Geometry check sheet. Reference: the model listing, model coordinates, mm. A direction names the side the tool comes from. Round coordinates to 2 decimals unless told otherwise and drop trailing zeros. Loops run counter-clockwise (first coordinate to the right, second up) from the corner with the lowest first, then second, coordinate; pieces in that order, holes last. Notation, with made-up numbers: (-13.5, 27.25) - (37.5, 27.25) arc R29 cw to (37.5, 62.25) - close; hole circle Ø9 at (30.5, -34). An arc over 180 degrees is marked (long way). Write item = value, one per line.
```python
from build123d import *

# Parameters (mm, degrees)
EXTRUDE_1_DEPTH             = 20
FILLET_1_R                  = 2
FILLET_2_R                  = 2
CUT_EXTRUDE_2_DEPTH         = 10
SKETCH_34_R                 = 3.25
CUT_EXTRUDE_3_DEPTH         = 6
HOLE_WIZARD_M4_2_D          = 3.3
HOLE_WIZARD_M4_2_DEPTH      = 4
SKETCH_38_W                 = 5
SKETCH_38_H                 = 10
CUT_EXTRUDE_4_DEPTH         = 11
SKETCH_40_W                 = 1.65
SKETCH_40_H                 = 8
HOLE_WIZARD_M4_3_AT_2_COUNT = 2
HOLE_WIZARD_M4_3_AT_2_PITCH = 10
CUT_EXTRUDE_5_DEPTH         = 4.5


with BuildPart() as part:
    # 草图1 → 凸台-拉伸1 (new body)
    with BuildSketch(Plane.XY):
        Polygon((0.020144186, -0.052366179), (0.016918395, 5.947632954), (-19.983081605, 5.947632954), (-20.000068427, 12.447632954), (0.03759791, 12.447632954), (0.03759791, 20.447632954), (-19.96240209, 20.447632954), (-11.597239053, 51.666846423), (-21.256497316, 54.255036874), (-30.315163894, 20.447632954), (-30.279663837, -0.052366179), align=None)
    extrude(amount=EXTRUDE_1_DEPTH)

    # 圆角1
    fillet_1_edges = [part.edges().sort_by_distance(p)[0] for p in [
        (-19.96240209, 20.447632954, 10),
    ]]
    fillet(fillet_1_edges, radius=FILLET_1_R)

    # 圆角2
    fillet_2_edges = [part.edges().sort_by_distance(p)[0] for p in [
        (-30.279663837, -0.052366179, 10),
    ]]
    fillet(fillet_2_edges, radius=FILLET_2_R)

    # 草图33 → 切除-拉伸2 (cut)
    with BuildSketch(Plane.XY.offset(20)):
        Polygon((-21.256497316, 54.255036874), (-11.597239053, 51.666846423), (-14.185429504, 42.00758816), (-23.844687767, 44.595778611), align=None)
    extrude(amount=-CUT_EXTRUDE_2_DEPTH, mode=Mode.SUBTRACT)

    # 草图34 → 切除-拉伸3 (cut)
    with BuildSketch(Plane(origin=(0, 0, 0), x_dir=(-1, 0, 0), z_dir=(0, 0, -1))):
        with Locations((17.72096341, 48.131312517)):
            Circle(SKETCH_34_R)
    extrude(amount=-CUT_EXTRUDE_3_DEPTH, mode=Mode.SUBTRACT)

    # M4 螺纹孔的螺纹孔钻头2
    with Locations(Plane(origin=(0, 0, 6), x_dir=(-1, 0, 0), z_dir=(0, 0, -1))):
        with Locations((17.72096341, 48.131312517)):
            Hole(HOLE_WIZARD_M4_2_D / 2, depth=HOLE_WIZARD_M4_2_DEPTH)

    # 草图38 → 切除-拉伸4 (cut)
    with BuildSketch(Plane(origin=(-23.737082949, 6.360332207, 0), x_dir=(0, 0, -1), z_dir=(0.965925826, -0.258819045, 0))):
        with Locations((-2.5, 41.904754985)):
            Rectangle(SKETCH_38_W, SKETCH_38_H)
    extrude(amount=-CUT_EXTRUDE_4_DEPTH, mode=Mode.SUBTRACT)

    # 草图40 → M4 螺纹孔的螺纹孔钻头3 (revolve, cut)
    with BuildSketch(Plane(origin=(-5.798619526, 12.447632954, 5), x_dir=(0, 0, -1), z_dir=(1, 0, 0))):
        with Locations((0.825, 4)):
            Rectangle(SKETCH_40_W, SKETCH_40_H)
    hole_wizard_m4_3 = revolve(axis=Axis((-5.798619526, 6.097632954, 5), (0, 1, 0)), mode=Mode.SUBTRACT)

    # M4 螺纹孔的螺纹孔钻头3 at 2: M4 螺纹孔的螺纹孔钻头3 ×2
    with Locations(*[(0, 0, i * HOLE_WIZARD_M4_3_AT_2_PITCH) for i in range(1, HOLE_WIZARD_M4_3_AT_2_COUNT)]):
        add(hole_wizard_m4_3, mode=Mode.SUBTRACT)

    # 草图41 → 切除-拉伸5 (cut)
    with BuildSketch(Plane.XZ.offset(-12.447632954)):
        with BuildLine():
            Line((-7.265759602, 12.1), (-4.331479451, 12.1))
            ThreePointArc((-4.331479451, 12.1), (-2.548619526, 15), (-4.331479451, 17.9))
            Line((-4.331479451, 17.9), (-7.265759602, 17.9))
            ThreePointArc((-7.265759602, 17.9), (-9.048619526, 15), (-7.265759602, 12.1))
        make_face()
        with BuildLine():
            Line((-7.265759602, 2.1), (-4.331479451, 2.1))
            ThreePointArc((-4.331479451, 2.1), (-2.548619526, 5), (-4.331479451, 7.9))
            Line((-4.331479451, 7.9), (-7.265759602, 7.9))
            ThreePointArc((-7.265759602, 7.9), (-9.048619526, 5), (-7.265759602, 2.1))
        make_face()
    extrude(amount=-CUT_EXTRUDE_5_DEPTH, mode=Mode.SUBTRACT)


solid = part.part
```
(1) Section check B-B (x = -18). Enter the section's corners in (y, z).
Answers follow:
outline = (-0.05, 0) - (5.95, 0) - (5.95, 20) - (-0.05, 20) - close; (12.45, 0) - (20.55, 0) - (20.55, 20) - (12.45, 20) - close; (27.77, 0) - (43.03, 0) - (43.03, 5) - (44.89, 5) - (44.89, 6) - (46.51, 6) - (46.51, 10) - (43.03, 10) - (43.03, 20) - (27.77, 20) - close; (49.76, 6) - (51.37, 6) - (51.37, 5) - (53.38, 5) - (53.38, 10) - (49.76, 10) - close
(2) Scan lines: L1, parallel to Z at x = -5, y = 13.5; L2, parallel to Y at x = -6, z = 9.75; L3, parallel to X at y = 18.65, z = 15. Record each from-to range of solid material in increasing order. Write a range as [from, to].
Answers follow:
L1 = [0, 2.1], [7.9, 12.1], [17.9, 20]
L2 = [-0.05, 5.95], [12.45, 20.45]
L3 = [-30.31, -7.45], [-4.15, 0.04]
(3) Mould release check, pull along Y, two halves, no side actions. Record for faces 5 (the flat face through (-6, 16.948, 13)), 6 (the flat face through (-19, 18, 20)), 7 (the flat face through (-16.359, 52.943, 7.465)): pulls with the +Y half, pulls with the -Y half, needs draft (parallel to the pull), parting line crosses it, or undercut.
Answers follow:
face_5 = undercut
face_6 = needs draft
face_7 = pulls with the +Y half
(4) Set-up check for faces 1 (the cylindrical face through (-6.91, 18.72, 6.22)), 2 (the flat face through (-14, 47, 5)), 3 (the cylindrical face through (-2.55, 14.67, 14.95)), 4 (the flat face through (-9, 20.448, 10)): record each of +Z, -Z, +X, -X, +Y, -Y from which the full face is reachable in a straight line by a thin tool's end or side.
Answers follow:
face_1 = +Y
face_2 = -Z, +X, +Y
face_3 = none
face_4 = +Z, -Z, +X
(5) Gauge pin test, flat ends, axial feed: pin 1 (5 mm diameter, centred on y = 30.5, z = 10.5, fed in from -X); pin 2 (2 mm diameter, centred on x = -17, z = 11.5, fed in from +Y); pin 3 (3 mm diameter, centred on x = -16, y = 49, fed in from -Z); pin 4 (3 mm diameter, centred on x = -17.72, y = 48.13, fed in from +Z). Record the tip position at first contact, or that the pin passes through.
Answers follow:
pin_1 = -28.29
pin_2 = 43.03
pin_3 = 5
pin_4 = through
(6) Section check A-A (z = 15). Enter the section's corners in (x, y).
Answers follow:
outline = (-30.32, 20.45) - (-30.28, 1.94) arc R2 ccw to (-28.28, -0.05) - (0.02, -0.05) - (0.02, 5.95) - (-19.98, 5.95) - (-20, 12.45) - (-9.05, 12.45) - (-9.05, 16.95) - (-7.45, 16.95) - (-7.45, 20.45) - (-17.36, 20.45) arc R2 cw to (-19.29, 22.97) - (-14.19, 42.01) - (-23.84, 44.6) - close; (-4.15, 16.95) - (-2.55, 16.95) - (-2.55, 12.45) - (0.04, 12.45) - (0.04, 20.45) - (-4.15, 20.45) - close
(7) Section check C-C (x = -22). Enter the section's corners in (y, z).
Answers follow:
outline = (-0.05, 0) - (44.1, 0) - (44.1, 5) - (51.48, 5) - (51.48, 10) - (44.1, 10) - (44.1, 20) - (-0.05, 20) - close
(8) Section check D-D (z = 2.75). Enter the section's corners in (x, y).
Answers follow:
outline = (-30.32, 20.45) - (-30.28, 1.94) arc R2 ccw to (-28.28, -0.05) - (0.02, -0.05) - (0.02, 5.95) - (-19.98, 5.95) - (-20, 12.45) - (-8.14, 12.45) - (-8.14, 16.95) - (-3.45, 16.95) - (-3.45, 12.45) - (0.04, 12.45) - (0.04, 20.45) - (-17.36, 20.45) arc R2 cw to (-19.29, 22.97) - (-14.19, 42.01) - (-23.84, 44.6) - close
